from build123d import *

# Parameters (mm, degrees)
SKETCH1_W           = 55
SKETCH1_H           = 34.740153272
BOSS_EXTRUDE1_DEPTH = 30
SKETCH3_W           = 41
SKETCH3_H           = 21.140153272
CUT_EXTRUDE1_DEPTH  = 28.87
SKETCH5_W           = 7
SKETCH5_H           = 4.2
CUT_EXTRUDE2_DEPTH  = 10
SKETCH6_R           = 2.1
SKETCH6_R_2         = 1.99312569
CUT_EXTRUDE3_DEPTH  = 7
SKETCH7_R           = 4
BOSS_EXTRUDE2_DEPTH = 12
CHAMFER1_SIZE       = 2


with BuildPart() as part:
    # Sketch1 → Boss-Extrude1 (new body)
    with BuildSketch(Plane(origin=(0, 0, 0), x_dir=(1, 0, 0), z_dir=(0, 1, 0))):
        with Locations((27.5, 17.370076636)):
            Rectangle(SKETCH1_W, SKETCH1_H)
    extrude(amount=BOSS_EXTRUDE1_DEPTH)

    # Sketch3 → Cut-Extrude1 (cut)
    with BuildSketch(Plane(origin=(0, 30, 0), x_dir=(1, 0, 0), z_dir=(0, 1, 0))):
        with Locations((27.5, 17.370076636)):
            Rectangle(SKETCH3_W, SKETCH3_H)
    extrude(amount=-CUT_EXTRUDE1_DEPTH, mode=Mode.SUBTRACT)

    # Sketch5 → Cut-Extrude2 (cut)
    with BuildSketch(Plane.ZY):
        with Locations((-17.690153272, 6.5)):
            Rectangle(SKETCH5_W, SKETCH5_H)
    extrude(amount=-CUT_EXTRUDE2_DEPTH, mode=Mode.SUBTRACT)

    # Sketch6 → Cut-Extrude3 (cut)
    with BuildSketch(Plane(origin=(0, 30, 0), x_dir=(1, 0, 0), z_dir=(0, 1, 0))):
        with Locations((3.5, 22.690153272)):
            Circle(SKETCH6_R)
        with Locations((3.5, 12.690153272)):
            Circle(SKETCH6_R)
        with Locations((51.5, 12.690153272)):
            Circle(SKETCH6_R)
        with Locations((51.5, 22.690153272)):
            Circle(SKETCH6_R_2)
    extrude(amount=-CUT_EXTRUDE3_DEPTH, mode=Mode.SUBTRACT)

    # Sketch7 → Boss-Extrude2 (add)
    with BuildSketch(Plane.XZ):
        with Locations((17.25, -17.690153272)):
            Circle(SKETCH7_R)
    extrude(amount=BOSS_EXTRUDE2_DEPTH)

    # Chamfer1
    chamfer1_edges = [part.edges().sort_by_distance(p)[0] for p in [
        (0, 15, -34.740153272),
        (55, 15, -34.740153272),
    ]]
    chamfer(chamfer1_edges, length=CHAMFER1_SIZE)


solid = part.part
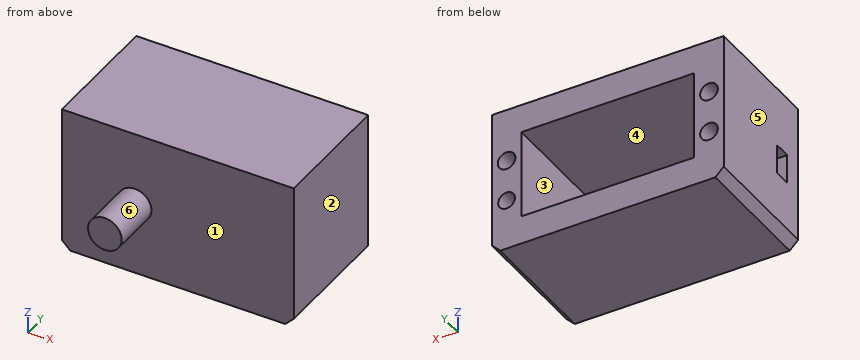
Source: CAD feature listing. Evaluate the final solid. Frame: model axes, mm. Face numbers are marked on the shaded views. A direction names the side the tool comes from. Round coordinates to 2 decimals unless told otherwise and drop trailing zeros. Loops run counter-clockwise (first coordinate to the right, second up) from the corner with the lowest first, then second, coordinate; pieces in that order, holes last.
Q1. Section A-A, the plane y = 10. Return loops of the section in (x, z), plus the area to 3 significant figures.
Q2. First-contact query: P1, Ø5.5, axis at x = 3.5, z = -12.69, coming from the -Y side; P2, Ø6, axis at y = -6.5, z = -27.5, coming from the +X side; P3, Ø1.2, axis at x = 52.5, z = -22.5, coming from the +Y side; P4, Ø5, axis at x = 39.5, y = 5.5, coming from the +Z side. Flat tips, straight axial feed; report the tip coordinate or a pass-through.
Q3. Ray query, line 1 (Z direction, x = 51.5, y = 27.5); line 2 (Z direction, x = 3.5, y = 25.25); line 3 (Z direction, x = 35, y = 3). Return the intervals inside material, ascending.
Q4. Access query for the marked faces 4, 5 and 6. Directions: +Z, -Z, +X, -X, +Y, -Y. A direction counts if a zero-diameter tool reaches every point of the face in a straight line with its end or side. Return the directions, or none.
Q5. Section C-C, the plane z = -9. Return loops of the section in (x, y), plus the area to 3 significant figures.
Q6. Mould query, pull axis X, two halves, no side actions, for the marked faces 1, 2 and 3. Classes: pulls with the +X half, pulls with the -X half, needs draft (parallel to the pull), parting line crosses it, or undercut.
Q7. Section B-B, the plane x = 3.5. Return loops of the section in (y, z), plus the area to 3 significant figures.
Q8. Section D-D, the plane x = 51.5. Return loops of the section in (y, z), plus the area to 3 significant figures.
Solutions:
1. outline: (0, -32.74) - (2, -34.74) - (53, -34.74) - (55, -32.74) - (55, 0) - (0, 0) - close; hole (7, -27.94) - (48, -27.94) - (48, -6.8) - (7, -6.8) - close
1. area: 1,040 mm2
2. P1: stops at y = 0
2. P2: passes through
2. P3: stops at y = 23
2. P4: stops at z = 0
3. line 1: z = -34.74 to -24.68, -20.7 to -14.79, -10.59 to 0
3. line 2: z = -34.74 to -24.79, -20.59 to -14.79, -10.59 to 0
3. line 3: z = -34.74 to -27.94, -6.8 to 0
4. face 4: +Y
4. face 5: +Z, -Z, -X, +Y, -Y
4. face 6: -Y
5. outline: (0, 0) - (55, 0) - (55, 30) - (48, 30) - (48, 1.13) - (7, 1.13) - (7, 30) - (0, 30) - close
5. area: 466 mm2
6. face 1: needs draft
6. face 2: pulls with the +X half
6. face 3: undercut
7. outline: (0, -34.74) - (30, -34.74) - (30, -24.79) - (23, -24.79) - (23, -20.59) - (30, -20.59) - (30, -14.79) - (23, -14.79) - (23, -10.59) - (30, -10.59) - (30, 0) - (0, 0) - close; hole (4.4, -21.19) - (8.6, -21.19) - (8.6, -14.19) - (4.4, -14.19) - close
7. area: 954 mm2
8. outline: (0, -34.74) - (30, -34.74) - (30, -24.68) - (23, -24.68) - (23, -20.7) - (30, -20.7) - (30, -14.79) - (23, -14.79) - (23, -10.59) - (30, -10.59) - (30, 0) - (0, 0) - close
8. area: 985 mm2
